Could you check a few things on this model? Use its own coordinates, in mm. A direction names the side the tool comes from. Round coordinates to 2 decimals unless told otherwise and drop trailing zeros. Loops run counter-clockwise (first coordinate to the right, second up) from the corner with the lowest first, then second, coordinate; pieces in that order, holes last. Notation, with made-up numbers: (64.25, 30) -> (85.25, 30) arc R20 ccw to (85.25, 55) -> close; hole circle Ø10 at (0, -31.75). An arc over 180 degrees is marked (long way). One line per item, written item: value.
```python
from build123d import *

# Parameters (mm, degrees)
BOSS_EXTRUDE1_DEPTH = 10
CHAMFER1_SIZE       = 4
CUT_EXTRUDE1_DEPTH  = 23.825424421


with BuildPart() as part:
    # Sketch1 → Boss-Extrude1 (new body)
    with BuildSketch(Plane.XY):
        Polygon((0, 0), (15, 0), (15, 14), (-10.5, 14), (-10.5, 0), (-6.5, 0), (-6.5, 10), (0, 10), align=None)
    extrude(amount=BOSS_EXTRUDE1_DEPTH)

    # Chamfer1
    chamfer1_edges = [part.edges().sort_by_distance(p)[0] for p in [
        (-10.5, 14, 5),
        (15, 14, 5),
        (-10.5, 0, 5),
    ]]
    chamfer(chamfer1_edges, length=CHAMFER1_SIZE - 0.0001)  # a hair under: the kernel refuses the full size

    # Sketch2 → Cut-Extrude1 (cut, through all)
    with BuildSketch(Plane.XY.offset(10)):
        Polygon((4.25, 0), (4.25, 1.5), (1.75, 1.5), (1.75, 4), (13.25, 4), (13.25, 1.5), (10.75, 1.5), (10.75, 0), align=None)
    extrude(amount=-CUT_EXTRUDE1_DEPTH, mode=Mode.SUBTRACT)


solid = part.part
```
(1) Please list where these lines run through material, in increasing order: L1, parallel to X at y = 7.25, z = 9; L2, parallel to X at y = 3.5, z = 4.75; L3, parallel to X at y = 2, z = 5.5.
Results below:
L1: x = -10.5 to -6.5, 0 to 15
L2: x = -10 to -6.5, 0 to 1.75, 13.25 to 15
L3: x = -8.5 to -6.5, 0 to 1.75, 13.25 to 15
(2) On a 3-axis mill with a long thin cutter (end or side, diameter ignored), from which of +Z, -Z, +X, -X, +Y, -Y can I reach the whole of each face in a straight line? I mean faces 1 (the face through (5, 9, 10)), 2 (the face through (3, 1.5, 5)), 3 (the face through (-6.5, 5, 5)). Say none if no direction works.
Results below:
face 1: +Z, +X, -X, +Y, -Y
face 2: +Z, -Z
face 3: +Z, -Z, -Y
(3) Imagine slicing it at C-C on y = 1. Write out the boundary of the cut face in (x, z), then the cut area to 3 significant figures.
Results below:
outline: (-7.5, 0) -> (-6.5, 0) -> (-6.5, 10) -> (-7.5, 10) -> close; (0, 0) -> (4.25, 0) -> (4.25, 10) -> (0, 10) -> close; (10.75, 0) -> (15, 0) -> (15, 10) -> (10.75, 10) -> close
area: 95.0 mm²
(4) Imagine slicing it at A-A on x = 2.75. Write out the boundary of the cut face in (y, z), then the cut area to 3 significant figures.
Results below:
outline: (0, 0) -> (1.5, 0) -> (1.5, 10) -> (0, 10) -> close; (4, 0) -> (14, 0) -> (14, 10) -> (4, 10) -> close
area: 115 mm²
(5) For pin 1 Ø2 at (x, z) = (-3.5, 4.5) entering from -Y; pin 2 Ø2 at (y, z) = (2.5, 3) entering from -X; pin 3 Ø1 at (x, y) = (12, 3) entering from +Z, each with a flat end and sliding along its axis, tell me the tip position at first contact or that it passes through.
Results below:
pin 1: stops at y = 10
pin 2: stops at x = -10
pin 3: passes through
(6) We'd pull the mould along Y, two halves only. Please class faces 4 (the face through (0, 5, 5)), 5 (the face through (13, 0, 5)), 6 (the face through (7, 4, 5)), 7 (the face through (-8.5, 12, 4.9)): +Y half, -Y half, draft (parallel to the pull), parting line (faces both ways), or undercut.
Results below:
face 4: draft
face 5: -Y half
face 6: undercut
face 7: +Y half
(7) Imagine slicing it at B-B on y = 5.5. Write out the boundary of the cut face in (x, z), then the cut area to 3 significant figures.
Results below:
outline: (-10.5, 0) -> (-6.5, 0) -> (-6.5, 10) -> (-10.5, 10) -> close; (0, 0) -> (15, 0) -> (15, 10) -> (0, 10) -> close
area: 190 mm²
